Can you work these out from the drawing? Everything is in mm from the part's minimum corner. Round coordinates to 2 decimals unless told otherwise and drop trailing zeros. Loops run counter-clockwise (first coordinate to the right, second up) from the corner with the lowest first, then second, coordinate; pieces in that order, holes last. Notation, with made-up numbers: (-14.5, 21) -> (22.5, 21) arc R16 ccw to (22.5, 33) -> close; hole circle Ø1 at (76, 71.5). An arc over 180 degrees is marked (long way). One line per item, written item: value.
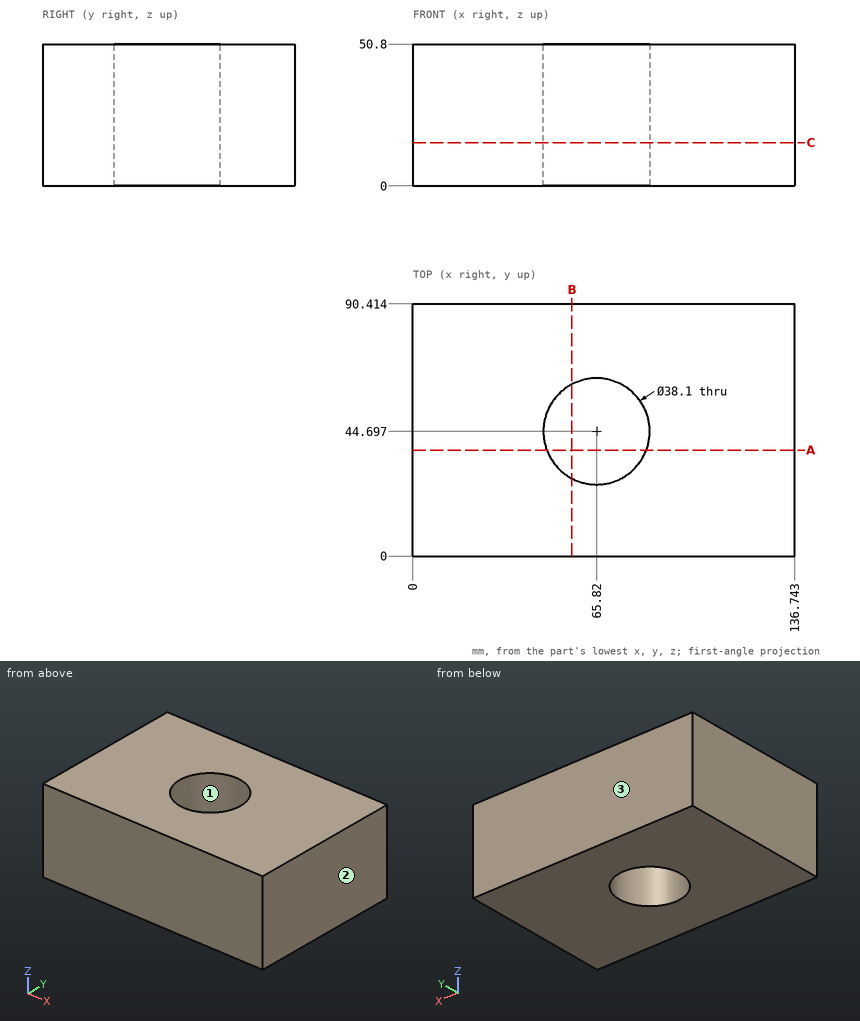
Item 1: I need wall thicknesses on line 1 (Y direction, x = 65, z = 9.5) (1 decimal); line 2 (X direction, y = 29.5, z = 36) (1 decimal); line 3 (X direction, y = 55.5, z = 30.5) (1 decimal). Which ranges of each line are inside material? Lowest first, please. Write a range as from..to.
Output:
line 1: y = 0..25.7, 63.7..90.4
line 2: x = 0..54.3, 77.3..136.7
line 3: x = 0..50.1, 81.5..136.7
Item 2: If we mould it in two halves opening along Y, with no side actions, what happens to the marked faces 1, 2 and 3? For each: released by +Y, released by -Y, zero draft, split by the parting line, or undercut.
Output:
face 1: undercut
face 2: zero draft
face 3: released by +Y
Item 3: If we section it at A-A on y = 38: List the corners of the cut face in (x, z) for me (1 decimal), plus the area to 3 significant figures.
Output:
outline: (0, 0) -> (48, 0) -> (48, 50.8) -> (0, 50.8) -> close; (83.7, 0) -> (136.7, 0) -> (136.7, 50.8) -> (83.7, 50.8) -> close
area: 5,130 mm²
Item 4: If we section it at C-C on z = 15.5: List the corners of the cut face in (x, y) for me.
Output:
outline: (0, 0) -> (136.74, 0) -> (136.74, 90.41) -> (0, 90.41) -> close; hole circle Ø38.1 at (65.82, 44.7)
Item 5: If we section it at B-B on x = 57: List the corners of the cut face in (y, z) for me.
Output:
outline: (0, 0) -> (27.81, 0) -> (27.81, 50.8) -> (0, 50.8) -> close; (61.58, 0) -> (90.41, 0) -> (90.41, 50.8) -> (61.58, 50.8) -> close
